```python
from build123d import *

# Parameters (mm, degrees)
SKETCH1_W                                            = 140
SKETCH1_H                                            = 50
BOSS_EXTRUDE1_DEPTH                                  = 10
CBORE_FOR_M6_HEXAGON_SOCKET_HEAD_CAP_SCR_D           = 6.6
CBORE_FOR_M6_HEXAGON_SOCKET_HEAD_CAP_SCR_CBORE_D     = 11
CBORE_FOR_M6_HEXAGON_SOCKET_HEAD_CAP_SCR_CBORE_DEPTH = 6.8
CBORE_FOR_M6_HEXAGON_SOCKET_HEAD_CAP_2_D             = 6.6
CBORE_FOR_M6_HEXAGON_SOCKET_HEAD_CAP_2_CBORE_D       = 11
CBORE_FOR_M6_HEXAGON_SOCKET_HEAD_CAP_2_CBORE_DEPTH   = 6.8
CHAMFER1_SIZE                                        = 5


with BuildPart() as part:
    # Sketch1 → Boss-Extrude1 (new body)
    with BuildSketch(Plane(origin=(0, 0, 0), x_dir=(1, 0, 0), z_dir=(0, 1, 0))):
        Rectangle(SKETCH1_W, SKETCH1_H)
    extrude(amount=BOSS_EXTRUDE1_DEPTH)

    # CBORE for M6 Hexagon socket head cap scr (through all)
    with Locations(Plane(origin=(0, 10, 0), x_dir=(1, 0, 0), z_dir=(0, 1, 0))):
        with Locations((-60, 15), (60, 15), (60, -15), (-60, -15)):
            CounterBoreHole(CBORE_FOR_M6_HEXAGON_SOCKET_HEAD_CAP_SCR_D / 2, CBORE_FOR_M6_HEXAGON_SOCKET_HEAD_CAP_SCR_CBORE_D / 2, CBORE_FOR_M6_HEXAGON_SOCKET_HEAD_CAP_SCR_CBORE_DEPTH)

    # CBORE for M6 Hexagon socket head cap 2 (through all)
    with Locations(Plane(origin=(0, 0, 0), x_dir=(-1, 0, 0), z_dir=(0, -1, 0))):
        with Locations((-40, 10), (-40, -15), (40, -15), (40, 10)):
            CounterBoreHole(CBORE_FOR_M6_HEXAGON_SOCKET_HEAD_CAP_2_D / 2, CBORE_FOR_M6_HEXAGON_SOCKET_HEAD_CAP_2_CBORE_D / 2, CBORE_FOR_M6_HEXAGON_SOCKET_HEAD_CAP_2_CBORE_DEPTH)

    # Chamfer1
    chamfer1_edges = [part.edges().sort_by_distance(p)[0] for p in [
        (70, 5, 25),
        (-70, 5, 25),
    ]]
    chamfer(chamfer1_edges, length=CHAMFER1_SIZE)


solid = part.part
```
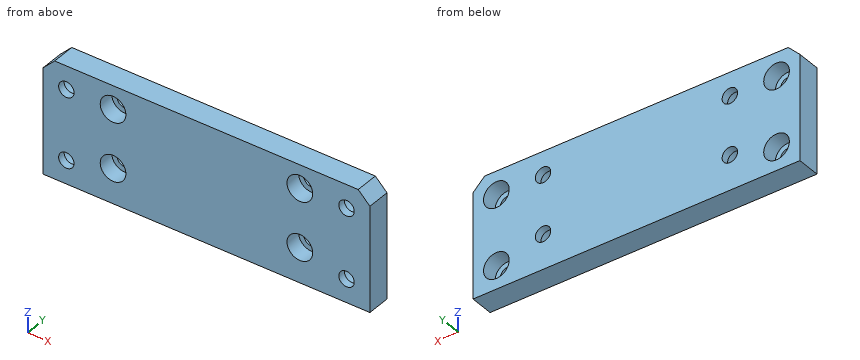
For this review, take the finished solid that the model builds, in its own axes (mm). Coordinates: 2 decimals unless noted, no trailing zeros. Order: outer loops, then holes, each group sorted by start corner. A loop starts at its lowest first (then second) coordinate and runs counter-clockwise, first axis right, second up. Notation, with made-up numbers: (-38.75, -17.75) - (-14.75, -17.75) arc R21 ccw to (-14.75, 16.25) - close; hole circle Ø1 at (41.25, 85.25). An arc over 180 degrees is marked (long way). Answer as a JSON object with one key per item and string values. Group by question number.
1. We need section D-D on x = 60.5. State the section outline as (y, z) points.
2. For probe 1 along Z at (x, y) = (60, 8.75); probe 2 along X at (y, z) = (6.25, 14.5); probe 3 along X at (y, z) = (9, 17.5), list the stretches that pass through material, from the lowest coordinate up.
3. We need section B-B on y = 8. Give the number of separate pieces and of enclosed holes in the cut face, then the cut area to 3 significant figures.
4. We need section A-A on x = -60. State the section outline as (y, z) points.
5. Clearance check with flat-ended pins moving along their axes: P1, Ø3.5, axis at x = 40.5, z = -8.5, coming from the -Y side; P2, Ø10, axis at x = 60, z = -15, coming from the +Y side. State where each tip first meets the part, or that it passes through.
Final values:
{
 "1": {"outline": "(0, -25) - (10, -25) - (10, -20.48) - (3.2, -20.48) - (3.2, -18.26) - (0, -18.26) - close; (0, -11.74) - (3.2, -11.74) - (3.2, -9.52) - (10, -9.52) - (10, 9.52) - (3.2, 9.52) - (3.2, 11.74) - (0, 11.74) - close; (0, 18.26) - (3.2, 18.26) - (3.2, 20.48) - (10, 20.48) - (10, 25) - (0, 25) - close"},
 "2": {"probe 1": "-25 to -20.5, -9.5 to 9.5, 20.5 to 25", "probe 2": "-70 to -65.48, -54.52 to -45.48, -34.52 to 34.52, 45.48 to 54.52, 65.48 to 70", "probe 3": "-70 to -64.9, -55.1 to -42.15, -37.85 to 37.85, 42.15 to 55.1, 64.9 to 70"},
 "3": {"separate pieces": "1", "enclosed holes": "8", "area": "6,460 mm²"},
 "4": {"outline": "(0, -25) - (10, -25) - (10, -20.5) - (3.2, -20.5) - (3.2, -18.3) - (0, -18.3) - close; (0, -11.7) - (3.2, -11.7) - (3.2, -9.5) - (10, -9.5) - (10, 9.5) - (3.2, 9.5) - (3.2, 11.7) - (0, 11.7) - close; (0, 18.3) - (3.2, 18.3) - (3.2, 20.5) - (10, 20.5) - (10, 25) - (0, 25) - close"},
 "5": {"P1": "y = 6.8", "P2": "y = 3.2"}
}
